Build history of the part. All positions in model axes, mm. Face numbers are marked on the shaded views. A direction names the side the tool comes from. Round coordinates to 2 decimals unless told otherwise and drop trailing zeros. Write each loop counter-clockwise with the first axis right and the second up, starting at its lowest first coordinate (ties: lowest second). Pieces come first, ordered by that corner, then holes.
from build123d import *

# Parameters (mm, degrees)
SKETCH1_W           = 30.4
SKETCH1_H           = 42
BOSS_EXTRUDE1_DEPTH = 1.8
SKETCH2_W           = 30.4
SKETCH2_H           = 1.4
BOSS_EXTRUDE2_DEPTH = 20
SKETCH3_R           = 1.5
CUT_EXTRUDE1_DEPTH  = 20
SKETCH4_R           = 3.875
SKETCH4_R_2         = 1
CUT_EXTRUDE2_DEPTH  = 20
SKETCH5_W           = 30.4
SKETCH5_H           = 2
BOSS_EXTRUDE3_DEPTH = 12.5
SKETCH6_R           = 10.4
CUT_EXTRUDE3_DEPTH  = 10


with BuildPart() as part:
    # Sketch1 → Boss-Extrude1 (new body)
    with BuildSketch(Plane(origin=(0, 0, 0), x_dir=(1, 0, 0), z_dir=(0, 1, 0))):
        Rectangle(SKETCH1_W, SKETCH1_H)
    extrude(amount=BOSS_EXTRUDE1_DEPTH)

    # Sketch2 → Boss-Extrude2 (add)
    with BuildSketch(Plane(origin=(0, 1.8, 0), x_dir=(1, 0, 0), z_dir=(0, 1, 0))):
        with Locations((0, 20.3)):
            Rectangle(SKETCH2_W, SKETCH2_H)
    extrude(amount=BOSS_EXTRUDE2_DEPTH)

    # Sketch3 → Cut-Extrude1 (cut)
    with BuildSketch(Plane(origin=(0, 1.8, 0), x_dir=(1, 0, 0), z_dir=(0, 1, 0))):
        with Locations(Location((12.5, 15.6, 0), (0, 0, 270))):
            Circle(SKETCH3_R)
        with Locations(Location((-12.5, 15.6, 0), (0, 0, 270))):
            Circle(SKETCH3_R)
        with Locations(Location((-12.5, -17, 0), (0, 0, 270))):
            Circle(SKETCH3_R)
        with Locations(Location((12.5, -17, 0), (0, 0, 270))):
            Circle(SKETCH3_R)
    extrude(amount=-CUT_EXTRUDE1_DEPTH, mode=Mode.SUBTRACT)

    # Sketch4 → Cut-Extrude2 (cut)
    with BuildSketch(Plane.XY.offset(-19.6)):
        with Locations((0, 14.58)):
            Circle(SKETCH4_R)
        with Locations((-7.75, 14.58)):
            Circle(SKETCH4_R_2)
        with Locations((7.75, 14.58)):
            Circle(SKETCH4_R_2)
        Polygon((-15.2, 16.4), (-9.8, 21.8), (-15.2, 21.8), align=None)
        Polygon((15.2, 16.4), (15.2, 21.8), (9.8, 21.8), align=None)
    extrude(amount=-CUT_EXTRUDE2_DEPTH, mode=Mode.SUBTRACT)

    # Sketch5 → Boss-Extrude3 (add)
    with BuildSketch(Plane(origin=(0, 1.8, 0), x_dir=(1, 0, 0), z_dir=(0, 1, 0))):
        with Locations((0, -7.283746966)):
            Rectangle(SKETCH5_W, SKETCH5_H)
    extrude(amount=BOSS_EXTRUDE3_DEPTH)

    # Sketch6 → Cut-Extrude3 (cut)
    with BuildSketch(Plane.XY.offset(8.283746966)):
        with Locations((0, 14.3)):
            Circle(SKETCH6_R)
    extrude(amount=-CUT_EXTRUDE3_DEPTH, mode=Mode.SUBTRACT)


solid = part.part
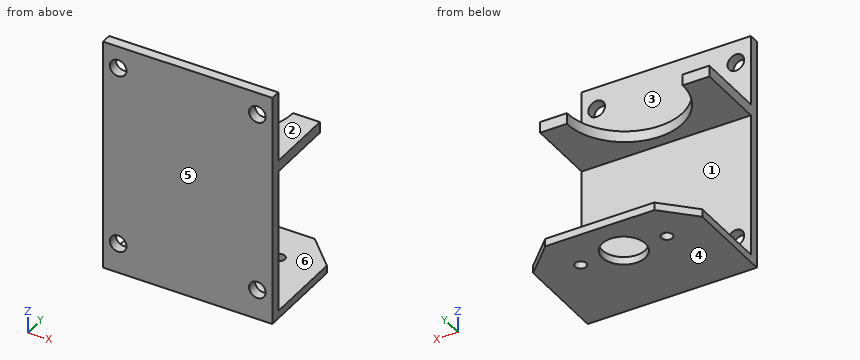
1) Mould opens along Z. For the marked faces 1, 2, 3 and 4 say: released by +Z, released by -Z, zero draft, split by the parting line, or undercut.
Results:
face 1: undercut
face 2: released by +Z
face 3: zero draft
face 4: released by -Z
2) Wall check: L1, parallel to Y at x = -7.75, z = -19.95; L2, parallel to X at y = 1.3, z = -15.6; L3, parallel to Z at x = 8, y = 6. Give the ranges that are in metal, low to high.
Results:
L1: y = 0 to 13.58, 15.58 to 21.8
L2: x = -15.2 to -14, -11 to 11, 14 to 15.2
L3: z = -21 to -19.6, 6.28 to 8.28
3) Slice it at C-C (y = 4.75). Write the cut outline in (x, z).
Results:
outline: (-15.2, -21) - (15.2, -21) - (15.2, -19.6) - (-15.2, -19.6) - close; (-15.2, 6.28) - (-4.12, 6.28) - (-4.12, 8.28) - (-15.2, 8.28) - close; (4.12, 6.28) - (15.2, 6.28) - (15.2, 8.28) - (4.12, 8.28) - close
4) Slice it at D-D (x = -7.75). Write the cut outline in (y, z).
Results:
outline: (0, -21) - (13.58, -21) - (13.58, -19.6) - (1.8, -19.6) - (1.8, 6.28) - (7.36, 6.28) - (7.36, 8.28) - (1.8, 8.28) - (1.8, 21) - (0, 21) - close; (15.58, -21) - (21.8, -21) - (21.8, -19.6) - (15.58, -19.6) - close
5) Slice it at A-A (x = 12.5). Write the cut outline in (y, z), plus the area to 3 significant figures.
Results:
outline: (0, -21) - (19.1, -21) - (19.1, -19.6) - (1.8, -19.6) - (1.8, -17.1) - (0, -17.1) - close; (0, -14.1) - (1.8, -14.1) - (1.8, 6.28) - (14.3, 6.28) - (14.3, 8.28) - (1.8, 8.28) - (1.8, 15.5) - (0, 15.5) - close; (0, 18.5) - (1.8, 18.5) - (1.8, 21) - (0, 21) - close
area: 114 mm2
6) Which spindle directions (+Z, -Z, +X, -X, +Y, -Y) get a long thin tool onto all of the face, cutting with end or side? Do the marked faces 5 and 6. Say none if no direction does.
Results:
face 5: +Z, -Z, +X, -X, -Y
face 6: +X, -X, +Y
7) Pin check, flat tips, straight feed: pin 1 Ø12 at (x, y) = (2.5, 15.5) entering from +Z; pin 2 Ø2.5 at (x, z) = (-12.5, -15.6) entering from +Y; pin 3 Ø1.5 at (x, z) = (-9, 5.5) entering from +Y; pin 4 Ø1 at (x, z) = (13, 7.5) entering from +Y. Stop position of each tip, or through.
Results:
pin 1: stops at z = -19.6
pin 2: passes through
pin 3: stops at y = 1.8
pin 4: stops at y = 14.3
8) Slice it at B-B (z = -15.6). Write the cut outline in (x, y).
Results:
outline: (-15.2, 0) - (-14, 0) - (-14, 1.8) - (-15.2, 1.8) - close; (-11, 0) - (11, 0) - (11, 1.8) - (-11, 1.8) - close; (14, 0) - (15.2, 0) - (15.2, 1.8) - (14, 1.8) - close
